Model file for the job. Use its own axes, mm. Round coordinates to 2 decimals unless told otherwise and drop trailing zeros. Order: outer loops, then holes, each group sorted by start corner. A loop starts at its lowest first (then second) coordinate and runs counter-clockwise, first axis right, second up. Notation, with made-up numbers: (22, 77) - (61, 77) arc R15 cw to (61, 97) - close; hole circle Ø8 at (-7.5, 57.5). An arc over 180 degrees is marked (long way). Write item = value, one per line.
```python
from build123d import *

# Parameters (mm, degrees)
EXTRUDE_1_DEPTH     = 4
SKETCH_4_OUTSIDE_W  = 19.022
SKETCH_4_OUTSIDE_H  = 13.522
SKETCH_4_OUTSIDE_R  = 4
CUT_EXTRUDE_1_DEPTH = 2.2
CUT_EXTRUDE_2_DEPTH = 6.8


with BuildPart() as part:
    # Эскиз1 → Бобышка-Вытянуть1 (new body, symmetric)
    with BuildSketch(Plane.XY):
        Polygon((4, 0), (-4, 0), (-4, -2.2), (-6.75, -2.2), (-6.75, -8), (6.75, -8), (6.75, -2.2), (4, -2.2), align=None)
    extrude(amount=EXTRUDE_1_DEPTH, both=True)

    # Эскиз3 → Отверстие обработанное метчиком M62 (revolve, cut)
    with BuildSketch(Plane(origin=(0, 0, 0), x_dir=(0, 0, 1), z_dir=(1, 0, 0))):
        Polygon((0, 0), (0, 8), (3.5, 8), (2.5, 7), (2.5, 1), (3.5, 0), align=None)
    revolve(axis=Axis((0, 6.35, 0), (0, -1, 0)), mode=Mode.SUBTRACT)

    # Эскиз4 outside → Вырез-Вытянуть1 (cut)
    with BuildSketch(Plane(origin=(0, 0, 0), x_dir=(1, 0, 0), z_dir=(0, 1, 0))):
        Rectangle(SKETCH_4_OUTSIDE_W, SKETCH_4_OUTSIDE_H)
        with Locations(Location((0, 0, 0), (0, 0, 270))):  # turned: the seam where the file's is
            Circle(SKETCH_4_OUTSIDE_R, mode=Mode.SUBTRACT)
    extrude(amount=-CUT_EXTRUDE_1_DEPTH, mode=Mode.SUBTRACT)

    # Эскиз5 → Вырез-Вытянуть2 (cut, through all)
    with BuildSketch(Plane(origin=(0, -2.2, 0), x_dir=(1, 0, 0), z_dir=(0, 1, 0))):
        with BuildLine():
            Line((-6.75, 0), (-6.75, 4))
            Line((-6.75, 4), (-5.437140793, 4))
            ThreePointArc((-5.437140793, 4), (-6.413392252, 2.104970267), (-6.75, 0))
        make_face()
        with BuildLine():
            Line((6.75, 0), (6.75, -4))
            Line((6.75, -4), (5.437140793, -4))
            ThreePointArc((5.437140793, -4), (6.413392252, -2.104970267), (6.75, 0))
        make_face()
    extrude(amount=-CUT_EXTRUDE_2_DEPTH, mode=Mode.SUBTRACT)

    # Вырез-По траектории1: sweep along a path in Эскиз7
    with BuildLine(Plane.XZ.offset(8)) as sweep_1_path:
        Line((0, 6.75), (-6.75, 6.75))
        Line((-6.75, 6.75), (-6.75, 0))
        ThreePointArc((-6.75, 0), (-4.772970773, -4.772970773), (0, -6.75))
        Line((0, -6.75), (6.75, -6.75))
        Line((6.75, -6.75), (6.75, 0))
        ThreePointArc((6.75, 0), (4.772970773, 4.772970773), (0, 6.75))
    # Эскиз6 → Вырез-По траектории1 (sweep, cut)
    with BuildSketch(Plane.XY.offset(4)):
        Polygon((-6.75, -4.7), (-6.75, -8), (-4, -8), align=None)
    sweep(path=sweep_1_path.line, transition=Transition.RIGHT, mode=Mode.SUBTRACT)


solid = part.part
```
1) Flat gauge pins, fed straight in: pin 1 Ø1.5 at (y, z) = (-5, 2.5) entering from +X; pin 2 Ø2 at (y, z) = (-4, -1.5) entering from -X. Where does each tip first touch, or does it go through?
Conclusion:
pin_1 = 6.5
pin_2 = -6.73
2) Mould opens along Z. For faces 1 (the face through (-3.905, -1.085, -0.867)), 2 (the face through (6.404, -3.432, 2.133)), 3 (the face through (2.44, -3.96, -0.54)), 4 (the face through (-5.36, -6.37, 1.97)) say: +Z half, -Z half, draft (parallel to the pull), parting line (faces both ways), or undercut.
Conclusion:
face_1 = parting line
face_2 = +Z half
face_3 = undercut
face_4 = draft
3) Wall check: line 1 along X through (y, z) = (-2.7, 0); line 2 along X through (y, z) = (-2.25, 2); line 3 along Z through (x, y) = (-2, -4.5). Give the ranges that are in metal, low to high.
Conclusion:
line_1 = -6.75 to -2.5, 2.5 to 6.75
line_2 = -6.75 to -1.5, 1.5 to 6.45
line_3 = -4 to -1.5, 1.5 to 4
4) Cut at A-A (y = -6.5). Write the cut outline in (x, z), and give its area (3 significant figures).
Conclusion:
outline = (-5.25, 0) arc R5.25 ccw to (-3.4, -4) - (5.25, -4) - (5.25, 0) arc R5.25 ccw to (3.4, 4) - (-5.25, 4) - close; hole circle Ø5 at (0, 0)
area = 59.8 mm^2
